from build123d import *

# Parameters (mm, degrees)
BODY_DEPTH         = 347
SK_FRONT_TAPS_R    = 2.5
FRONT_TAPS_DEPTH   = 16
SK_PORTS_R         = 4.283
PORTS_DEPTH        = 10
SK_BACK_PLATE_R    = 15
BACK_PLATE_DEPTH   = 4
FRONT_START        = -10
SK_FRONT_PLATE_R   = 15
FRONT_PLATE_DEPTH  = 10
SK_ROD_HOLDER_R    = 14
ROD_HOLDER_DEPTH   = 18
SK_ROD_R           = 6
ROD_DEPTH          = 730
SK_ROD_THREAD_R    = 4.4
ROD_THREAD_DEPTH   = 22
ROD_START          = -5
ROD_FLATS_DEPTH    = 5
SENSOR_START       = -631.6
SK_SENSOR_SLOT_W   = 6.8
SK_SENSOR_SLOT_H   = 5
SK_SENSOR_SLOT_W_2 = 5
SK_SENSOR_SLOT_H_2 = 6.8
SENSOR_SLOT_DEPTH  = 631.6
FRONT_CUT_REACH    = 669.559
SK_FRONT_CUT_W     = 21.8
SK_FRONT_CUT_H     = 5
SK_FRONT_CUT_W_2   = 5
SK_FRONT_CUT_H_2   = 21.8
BACK_CUT_REACH     = 723.502
SK_BACK_CUT_W      = 21.8
SK_BACK_CUT_H      = 5
SK_BACK_CUT_W_2    = 5
SK_BACK_CUT_H_2    = 21.8
ROD_NUT_DEPTH      = 5


with BuildPart() as part:
    # sk Body → Body (new, symmetric)
    with BuildSketch(Plane.XY):
        with BuildLine():
            Line((-16.25, 22.5), (16.25, 22.5))
            ThreePointArc((16.25, 22.5), (20.669417382, 20.669417382), (22.5, 16.25))
            Line((22.5, 16.25), (22.5, -16.25))
            ThreePointArc((22.5, -16.25), (20.669417382, -20.669417382), (16.25, -22.5))
            Line((16.25, -22.5), (-16.25, -22.5))
            ThreePointArc((-16.25, -22.5), (-20.669417382, -20.669417382), (-22.5, -16.25))
            Line((-22.5, -16.25), (-22.5, 16.25))
            ThreePointArc((-22.5, 16.25), (-20.669417382, 20.669417382), (-16.25, 22.5))
        make_face()
    extrude(amount=BODY_DEPTH, both=True)

    # sk Front Taps → Front Taps (cut)
    with BuildSketch(Plane.XY.offset(347)):
        with Locations((16.25, 16.25)):
            Circle(SK_FRONT_TAPS_R)
        with Locations((-16.25, 16.25)):
            Circle(SK_FRONT_TAPS_R)
        with Locations((-16.25, -16.25)):
            Circle(SK_FRONT_TAPS_R)
        with Locations((16.25, -16.25)):
            Circle(SK_FRONT_TAPS_R)
    front_taps = extrude(amount=-FRONT_TAPS_DEPTH, mode=Mode.SUBTRACT)

    # Back Taps: Front Taps across plane
    add(front_taps.mirror(Plane.XY), mode=Mode.SUBTRACT)

    # sk Ports → Ports (cut)
    with BuildSketch(Plane(origin=(22.5, 0, 0), x_dir=(0, 0, -1), z_dir=(1, 0, 0))):
        with Locations((-331.4, -6)):
            Circle(SK_PORTS_R)
        with Locations((331.4, 5.2)):
            Circle(SK_PORTS_R)
    extrude(amount=-PORTS_DEPTH, mode=Mode.SUBTRACT)

    # sk Back Plate → Back Plate (add)
    with BuildSketch(Plane(origin=(0, 0, -347), x_dir=(-1, 0, 0), z_dir=(0, 0, -1))):
        Circle(SK_BACK_PLATE_R)
    extrude(amount=BACK_PLATE_DEPTH)

    # sk Front Plate → Front Plate (add)
    with BuildSketch(Plane(origin=(0, 0, 347), x_dir=(-1, 0, 0), z_dir=(0, 0, -1)).offset(FRONT_START)):
        Circle(SK_FRONT_PLATE_R)
    extrude(amount=FRONT_PLATE_DEPTH)

    # sk Rod Holder → Rod Holder (add)
    with BuildSketch(Plane(origin=(0, 0, 347), x_dir=(-1, 0, 0), z_dir=(0, 0, -1))):
        Circle(SK_ROD_HOLDER_R)
    extrude(amount=-ROD_HOLDER_DEPTH)

    # sk Rod → Rod (add)
    with BuildSketch(Plane(origin=(0, 0, -347), x_dir=(-1, 0, 0), z_dir=(0, 0, -1))):
        Circle(SK_ROD_R)
    extrude(amount=-ROD_DEPTH)

    # sk Rod Thread → Rod Thread (add)
    with BuildSketch(Plane.XY.offset(383)):
        with Locations(Location((0, 0, 0), (0, 0, 180))):
            Circle(SK_ROD_THREAD_R)
    extrude(amount=ROD_THREAD_DEPTH)

    # sk Rod Flats → Rod Flats (cut)
    with BuildSketch(Plane.XY.offset(383).offset(ROD_START)):
        with BuildLine():
            Line((-5, 3.31662479), (-5, -3.31662479))
            ThreePointArc((-5, -3.31662479), (-6, 0), (-5, 3.31662479))
        make_face()
        with BuildLine():
            Line((5, 3.31662479), (5, -3.31662479))
            ThreePointArc((5, -3.31662479), (6, 0), (5, 3.31662479))
        make_face()
    extrude(amount=ROD_FLATS_DEPTH, mode=Mode.SUBTRACT)

    # sk Sensor Slot → Sensor Slot (cut)
    with BuildSketch(Plane.XY.offset(315.8).offset(SENSOR_START)):
        with Locations((-7.5, 20)):
            Rectangle(SK_SENSOR_SLOT_W, SK_SENSOR_SLOT_H)
        with Locations((7.5, 20)):
            Rectangle(SK_SENSOR_SLOT_W, SK_SENSOR_SLOT_H)
        with Locations((7.5, -20)):
            Rectangle(SK_SENSOR_SLOT_W, SK_SENSOR_SLOT_H)
        with Locations((-7.5, -20)):
            Rectangle(SK_SENSOR_SLOT_W, SK_SENSOR_SLOT_H)
        with Locations((-20, -7.5)):
            Rectangle(SK_SENSOR_SLOT_W_2, SK_SENSOR_SLOT_H_2)
        with Locations((-20, 7.5)):
            Rectangle(SK_SENSOR_SLOT_W_2, SK_SENSOR_SLOT_H_2)
    extrude(amount=SENSOR_SLOT_DEPTH, mode=Mode.SUBTRACT)

    # sk Front Cut → Front Cut (cut, up to next)
    with BuildSketch(Plane.XY.offset(315.8), mode=Mode.PRIVATE) as front_cut_sk1:
        with Locations((0, 20)):
            Rectangle(SK_FRONT_CUT_W, SK_FRONT_CUT_H)
    front_cut_tool1 = extrude(front_cut_sk1.sketch, amount=FRONT_CUT_REACH, mode=Mode.PRIVATE) & part.part
    # sk Front Cut → Front Cut (cut, up to next)
    with BuildSketch(Plane.XY.offset(315.8), mode=Mode.PRIVATE) as front_cut_sk2:
        with Locations((-20, 0)):
            Rectangle(SK_FRONT_CUT_W_2, SK_FRONT_CUT_H_2)
    front_cut_tool2 = extrude(front_cut_sk2.sketch, amount=FRONT_CUT_REACH, mode=Mode.PRIVATE) & part.part
    # sk Front Cut → Front Cut (cut, up to next)
    with BuildSketch(Plane.XY.offset(315.8), mode=Mode.PRIVATE) as front_cut_sk3:
        with Locations((0, -20)):
            Rectangle(SK_FRONT_CUT_W, SK_FRONT_CUT_H)
    front_cut_tool3 = extrude(front_cut_sk3.sketch, amount=FRONT_CUT_REACH, mode=Mode.PRIVATE) & part.part
    add(front_cut_tool1.solids().sort_by_distance((0, 20, 315.8))[0], mode=Mode.SUBTRACT)
    add(front_cut_tool2.solids().sort_by_distance((-20, 0, 315.8))[0], mode=Mode.SUBTRACT)
    add(front_cut_tool3.solids().sort_by_distance((0, -20, 315.8))[0], mode=Mode.SUBTRACT)

    # sk Back Cut → Back Cut (cut, up to next)
    with BuildSketch(Plane(origin=(0, 0, -315.8), x_dir=(-1, 0, 0), z_dir=(0, 0, -1)), mode=Mode.PRIVATE) as back_cut_sk1:
        with Locations((0, 20)):
            Rectangle(SK_BACK_CUT_W, SK_BACK_CUT_H)
    back_cut_tool1 = extrude(back_cut_sk1.sketch, amount=BACK_CUT_REACH, mode=Mode.PRIVATE) & part.part
    # sk Back Cut → Back Cut (cut, up to next)
    with BuildSketch(Plane(origin=(0, 0, -315.8), x_dir=(-1, 0, 0), z_dir=(0, 0, -1)), mode=Mode.PRIVATE) as back_cut_sk2:
        with Locations((20, 0)):
            Rectangle(SK_BACK_CUT_W_2, SK_BACK_CUT_H_2)
    back_cut_tool2 = extrude(back_cut_sk2.sketch, amount=BACK_CUT_REACH, mode=Mode.PRIVATE) & part.part
    # sk Back Cut → Back Cut (cut, up to next)
    with BuildSketch(Plane(origin=(0, 0, -315.8), x_dir=(-1, 0, 0), z_dir=(0, 0, -1)), mode=Mode.PRIVATE) as back_cut_sk3:
        with Locations((0, -20)):
            Rectangle(SK_BACK_CUT_W, SK_BACK_CUT_H)
    back_cut_tool3 = extrude(back_cut_sk3.sketch, amount=BACK_CUT_REACH, mode=Mode.PRIVATE) & part.part
    add(back_cut_tool1.solids().sort_by_distance((0, 20, -315.8))[0], mode=Mode.SUBTRACT)
    add(back_cut_tool2.solids().sort_by_distance((-20, 0, -315.8))[0], mode=Mode.SUBTRACT)
    add(back_cut_tool3.solids().sort_by_distance((0, -20, -315.8))[0], mode=Mode.SUBTRACT)

    # sk Rod Nut → Rod Nut (add)
    with BuildSketch(Plane.XY.offset(385)):
        Polygon((0, -9.237604307), (8, -4.618802154), (8, 4.618802154), (0, 9.237604307), (-8, 4.618802154), (-8, -4.618802154), align=None)
    extrude(amount=ROD_NUT_DEPTH)


solid = part.part
Source: CAD feature listing. Evaluate the final solid. Frame: model axes, mm. A direction names the side the tool comes from. Coordinates: 2 decimals unless noted, no trailing zeros. One line per item, written item: value. Start each with the question number.
1. Ray query, L1, parallel to Y at x = -16, z = 336; L2, parallel to Y at x = -20, z = -263.5. Return the intervals inside material, ascending.
2. Contact query for flat-ended pins moving along their axis: P1, Ø3, axis at x = -5.5, y = 17.5, coming from the -Z side; P2, Ø2.5, axis at x = 16.5, y = -17, coming from the -Z side; P3, Ø1, axis at x = -9, z = -65.5, coming from the -Y side; P4, Ø10, axis at y = 17, z = -85, coming from the -X side. Output: stop coordinate, or through.
3. Mould query, pull axis Y, two halves, no side actions, for faces 6 (the flat face through (15.3, 0.3, -347)), 7 (the cylindrical face through (6, 0, 374)), 8 (the flat face through (-17.5, 5, -5)). Classes: pulls with the +Y half, pulls with the -Y half, needs draft (parallel to the pull), parting line crosses it, or undercut.
4. Set-up query: faces 1 (the flat face through (-4, -4, 390)), 2 (the flat face through (22.5, 0, 5)), 3 (the flat face through (-4, -4, 385)), 4 (the flat face through (0, 0, -351)), 5 (the cylindrical face through (14.985, 0.66, -348.972)). Return all of +Z, -Z, +X, -X, +Y, -Y with unobstructed straight access to the full face (end or side cutting, diameter ignored); none if empty.
Verdict:
1. L1: y = -22.5 to -18.74, -13.76 to 13.76, 18.74 to 22.5
1. L2: y = -21.25 to -10.9, -4.1 to 4.1, 10.9 to 21.25
2. P1: stops at z = -347
2. P2: stops at z = -331
2. P3: stops at y = -17.5
2. P4: stops at x = -22.5
3. face 6: needs draft
3. face 7: parting line crosses it
3. face 8: undercut
4. face 1: +Z
4. face 2: +Z, -Z, +X, +Y, -Y
4. face 3: none
4. face 4: -Z, +X, -X, +Y, -Y
4. face 5: -Z
